Can you work these out from the model? Positions are in its coordinate system, mm. A direction names the side the tool comes from. Coordinates: 2 decimals unless noted, no trailing zeros. Loops run counter-clockwise (first coordinate to the right, second up) from the corner with the lowest first, then second, coordinate; pieces in that order, holes last.
```python
from build123d import *

# Parameters (mm, degrees)
CROQUIS1_W              = 200
CROQUIS1_H              = 80
SALIENTE_EXTRUIR1_DEPTH = 2.4
CROQUIS2_R              = 11
CORTAR_EXTRUIR1_DEPTH   = 108.730032953
CROQUIS3_R              = 3.25
CORTAR_EXTRUIR2_DEPTH   = 108.730032953
CORTAR_EXTRUIR3_DEPTH   = 2.4
CROQUIS7_W              = 64.4
CROQUIS7_H              = 56.4
CORTAR_EXTRUIR4_DEPTH   = 108.730032953
CROQUIS8_R              = 2.5
CORTAR_EXTRUIR5_DEPTH   = 108.730032953
REDONDEO1_R             = 5
REDONDEO2_R             = 5


with BuildPart() as part:
    # Croquis1 → Saliente-Extruir1 (new body)
    with BuildSketch(Plane.XY):
        Rectangle(CROQUIS1_W, CROQUIS1_H)
    extrude(amount=SALIENTE_EXTRUIR1_DEPTH)

    # Croquis2 → Cortar-Extruir1 (cut, through all)
    with BuildSketch(Plane.XY.offset(2.4)):
        Circle(CROQUIS2_R)
    extrude(amount=-CORTAR_EXTRUIR1_DEPTH, mode=Mode.SUBTRACT)

    # Croquis3 → Cortar-Extruir2 (cut, through all)
    with BuildSketch(Plane.XY.offset(2.4)):
        with Locations((20, 20)):
            Circle(CROQUIS3_R)
        with Locations((-20, 20)):
            Circle(CROQUIS3_R)
        with Locations((-20, -20)):
            Circle(CROQUIS3_R)
        with Locations((20, -20)):
            Circle(CROQUIS3_R)
    extrude(amount=-CORTAR_EXTRUIR2_DEPTH, mode=Mode.SUBTRACT)

    # Croquis4 → Cortar-Extruir3 (cut)
    with BuildSketch(Plane.XY.offset(2.4)):
        with BuildLine():
            Line((-62, 20), (-52, 20))
            ThreePointArc((-52, 20), (-32, 0), (-52, -20))
            Line((-52, -20), (-62, -20))
            ThreePointArc((-62, -20), (-82, 0), (-62, 20))
        make_face()
        with BuildLine():
            Line((-85.55, 26.05), (-75.55, 26.05))
            ThreePointArc((-75.55, 26.05), (-73.05, 23.55), (-75.55, 21.05))
            Line((-75.55, 21.05), (-85.55, 21.05))
            ThreePointArc((-85.55, 21.05), (-88.05, 23.55), (-85.55, 26.05))
        make_face()
        with BuildLine():
            Line((-28.45, 21.05), (-38.45, 21.05))
            ThreePointArc((-38.45, 21.05), (-40.95, 23.55), (-38.45, 26.05))
            Line((-38.45, 26.05), (-28.45, 26.05))
            ThreePointArc((-28.45, 26.05), (-25.95, 23.55), (-28.45, 21.05))
        make_face()
        with BuildLine():
            Line((-28.45, -26.05), (-38.45, -26.05))
            ThreePointArc((-38.45, -26.05), (-40.95, -23.55), (-38.45, -21.05))
            Line((-38.45, -21.05), (-28.45, -21.05))
            ThreePointArc((-28.45, -21.05), (-25.95, -23.55), (-28.45, -26.05))
        make_face()
        with BuildLine():
            Line((-85.55, -21.05), (-75.55, -21.05))
            ThreePointArc((-75.55, -21.05), (-73.05, -23.55), (-75.55, -26.05))
            Line((-75.55, -26.05), (-85.55, -26.05))
            ThreePointArc((-85.55, -26.05), (-88.05, -23.55), (-85.55, -21.05))
        make_face()
    extrude(amount=-CORTAR_EXTRUIR3_DEPTH, mode=Mode.SUBTRACT)

    # Croquis7 → Cortar-Extruir4 (cut, through all)
    with BuildSketch(Plane.XY.offset(2.4)):
        with Locations((57, 0)):
            Rectangle(CROQUIS7_W, CROQUIS7_H)
    extrude(amount=-CORTAR_EXTRUIR4_DEPTH, mode=Mode.SUBTRACT)

    # Croquis8 → Cortar-Extruir5 (cut, through all)
    with BuildSketch(Plane.XY.offset(2.4)):
        with Locations((39, 34)):
            Circle(CROQUIS8_R)
        with Locations((75, 34)):
            Circle(CROQUIS8_R)
        with Locations((39, -34)):
            Circle(CROQUIS8_R)
        with Locations((75, -34)):
            Circle(CROQUIS8_R)
    extrude(amount=-CORTAR_EXTRUIR5_DEPTH, mode=Mode.SUBTRACT)

    # Redondeo1
    redondeo1_edges = [part.edges().sort_by_distance(p)[0] for p in [
        (89.2, 28.2, 1.2),
        (89.2, -28.2, 1.2),
        (24.8, -28.2, 1.2),
        (24.8, 28.2, 1.2),
    ]]
    fillet(redondeo1_edges, radius=REDONDEO1_R)

    # Redondeo2
    redondeo2_edges = [part.edges().sort_by_distance(p)[0] for p in [
        (100, -40, 1.2),
        (-100, -40, 1.2),
        (-100, 40, 1.2),
        (100, 40, 1.2),
    ]]
    fillet(redondeo2_edges, radius=REDONDEO2_R)


solid = part.part
```
Item 1: Suppose I cut it at B-B, the plane x = -54.5. Please give me the cut outline in (y, z).
Results are:
outline: (-40, 0) - (-20, 0) - (-20, 2.4) - (-40, 2.4) - close; (20, 0) - (40, 0) - (40, 2.4) - (20, 2.4) - close
Item 2: Suppose I cut it at D-D, the plane x = 20. Please give me the cut outline in (y, z).
Results are:
outline: (-40, 0) - (-23.25, 0) - (-23.25, 2.4) - (-40, 2.4) - close; (-16.75, 0) - (16.75, 0) - (16.75, 2.4) - (-16.75, 2.4) - close; (23.25, 0) - (40, 0) - (40, 2.4) - (23.25, 2.4) - close
Item 3: I need wall thicknesses on line 1 along Y through (x, z) = (75, 0.7); line 2 along Y through (x, z) = (-20, 1.2); line 3 along X through (y, z) = (-35.5, 0.45). Which ranges of each line are inside material? Lowest first, please.
Results are:
line 1: y = -40 to -36.5, -31.5 to -28.2, 28.2 to 31.5, 36.5 to 40
line 2: y = -40 to -23.25, -16.75 to 16.75, 23.25 to 40
line 3: x = -99.97 to 37, 41 to 73, 77 to 99.97
Item 4: Suppose I cut it at A-A, the plane x = 75. Please give me the cut outline in (y, z), plus the area to 3 significant figures.
Results are:
outline: (-40, 0) - (-36.5, 0) - (-36.5, 2.4) - (-40, 2.4) - close; (-31.5, 0) - (-28.2, 0) - (-28.2, 2.4) - (-31.5, 2.4) - close; (28.2, 0) - (31.5, 0) - (31.5, 2.4) - (28.2, 2.4) - close; (36.5, 0) - (40, 0) - (40, 2.4) - (36.5, 2.4) - close
area: 32.6 mm2
Item 5: Suppose I cut it at C-C, the plane y = 0. Please give me the cut outline in (x, z), plus the area to 3 significant figures.
Results are:
outline: (-100, 0) - (-82, 0) - (-82, 2.4) - (-100, 2.4) - close; (-32, 0) - (-11, 0) - (-11, 2.4) - (-32, 2.4) - close; (11, 0) - (24.8, 0) - (24.8, 2.4) - (11, 2.4) - close; (89.2, 0) - (100, 0) - (100, 2.4) - (89.2, 2.4) - close
area: 153 mm2
Item 6: On a 3-axis mill with a long thin cutter (end or side, diameter ignored), from which of +Z, -Z, +X, -X, +Y, -Y can I reach the whole of each face in a straight line? I mean faces 1 (the face through (-24, 1, 2.4)), 2 (the face through (87.7, -26.77, 1.18)). Say none if no direction works.
Results are:
face 1: +Z, +X, -X, +Y, -Y
face 2: +Z, -Z
Item 7: We'd pull the mould along X, two halves only. Please class faces 3 (the face through (98, 39, 1)), 4 (the face through (16.753, 20.143, 1.217)), 5 (the face through (-24, 1, 0)): +X half, -X half, draft (parallel to the pull), parting line (faces both ways), or undercut.
Results are:
face 3: +X half
face 4: undercut
face 5: draft
Item 8: I'm going to push a flat-ended pin straight in: P1, Ø6, axis at x = 20, y = 20, coming from the -Z side. Where does the tip first touch, or does it pass through?
Results are:
P1: passes through
